Verification items for the finished model (mm, model axes). A direction names the side the tool comes from. Round coordinates to 2 decimals unless told otherwise and drop trailing zeros. Write each loop counter-clockwise with the first axis right and the second up, starting at its lowest first coordinate (ties: lowest second). Pieces come first, ordered by that corner, then holes. Notation, with made-up numbers: (-26.75, 80) -> (-1.75, 80) arc R36 cw to (-1.75, 119) -> close; hole circle Ø7 at (15.5, 23). An arc over 180 degrees is marked (long way). Answer as a JSON object with one key per item and string values. Group by question number.
(1) Scan lines: L1, parallel to X at y = -2.5, z = 265.5; L2, parallel to Z at x = 24, y = 9; L3, parallel to X at y = 18.5, z = 102. Record each from-to range of solid material in increasing order. Write a range as from..to.
(2) Set-up check for faces 1 (the face through (-5, -3.962, 267)), 2 (the face through (12.7, 0, 260)), 3 (the face through (-12.7, 0, 260)): record each of +Z, -Z, +X, -X, +Y, -Y from which the full face is reachable in a straight line by a thin tool's end or side.
(3) Sectioned sample at C-C on z = 104.5. Record the cut outline in (x, y), and give its area (3 significant figures).
(4) Sectioned sample at D-D on x = -15.5. Record the cut outline in (y, z), and give its area (3 significant figures).
(5) Sectioned sample at B-B on y = 0. Record the cut outline in (x, z).
(6) Gauge pin test, flat ends, axial feed: pin 1 Ø4 at (y, z) = (1, 262) entering from +X; pin 2 Ø3 at (y, z) = (11, 186) entering from +X; pin 3 Ø1.5 at (y, z) = (-1, 199.5) entering from +X. Record the tip position at first contact, or that the pin passes through.
(7) Sectioned sample at A-A on x = 0. Record the cut outline in (y, z), and give its area (3 significant figures).
(8) Draft check along X on faces 4 (the face through (5, 3.962, 267)), 5 (the face through (-0.279, 0.055, 279.397)), 6 (the face through (4.775, 0, 260)), 7 (the face through (-4.775, 0, 260)). Enter one of: released by +X, released by -X, zero draft, split by the parting line, or undercut.
Autodesk Inventor part; units mm, degrees
ref_plane "YZ Plane" through (0, 0, 0) normal (1, 0, 0) x (0, 1, 0)
ref_plane "XZ Plane" through (0, 0, 0) normal (0, 1, 0) x (-1, 0, 0)
ref_plane "XY Plane" through (0, 0, 0) normal (0, 0, 1) x (1, 0, 0)
sketch "Sketch1" plane through (0, 0, 0) normal (0, 0, 1) x (1, 0, 0)
  circle A0 centre (0, 0) radius 31.2674
  dimension "d0" = 62.5348
extrude "Extrusion1" add sketch "Sketch1" along normal blind 254
sketch "Sketch2" plane through (0, 0, 254) normal (0, 0, 1) x (1, 0, 0)
  circle A0 centre (0, 0) radius 31.2674
  line L0 (-12.7, 3.9624) -> (12.7, 3.9624)
  line L1 (12.7, 3.9624) -> (12.7, -3.9624)
  line L2 (12.7, -3.9624) -> (-12.7, -3.9624)
  line L3 (-12.7, -3.9624) -> (-12.7, 3.9624)
  dimension "d3" = 7.9248
  dimension "d4" = 3.9624
  dimension "d5" = 12.7
  dimension "d6" = 12.7
extrude "Extrusion2" add sketch "Sketch2" along normal blind 25.4 contours L0 L1 L2 L3
sketch "Sketch3" plane through (-12.7, 3.9624, 254) normal (0, 1, 0) x (1, 0, 0)
  line L0 (0, 0) -> (25.4, 0)
  line L1 (0, 0) -> (0, -25.4)
  line L2 (25.4, -25.4) -> (0, -25.4)
  line L3 (25.4, 0) -> (25.4, -25.4)
  arc A0 (0, -12.7) -> (25.4, -12.7) centre (12.7, -12.7) ccw
  line L4 (7.9248, 0) -> (7.9248, -12.7)
  line L5 (17.4752, 0) -> (17.4752, -12.7)
  arc A1 (7.9248, -12.7) -> (17.4752, -12.7) centre (12.7, -12.7) ccw
  point P0 (12.7, 254)
  dimension "d9" = 7.9248
extrude "Extrusion3" cut sketch "Sketch3" against normal blind 25.4 contours L0 L5 A1 L4 | A0 L2 L1 | A0 L3 L2
properties part number "Spring End"
Computed values:
{
 "1": {"L1": "-12.7..-4.78, 4.78..12.7", "L2": "0..254", "L3": "-25.21..25.21"},
 "2": {"face 1": "+Z, +X, -X, -Y", "face 2": "+Z, +X, +Y, -Y", "face 3": "+Z, -X, +Y, -Y"},
 "3": {"outline": "circle Ø62.53 at (0, 0)", "area": "3,070 mm2"},
 "4": {"outline": "(-27.16, 0) -> (27.16, 0) -> (27.16, 254) -> (-27.16, 254) -> close", "area": "13,800 mm2"},
 "5": {"outline": "(-31.27, 0) -> (31.27, 0) -> (31.27, 254) -> (12.7, 254) -> (12.7, 266.7) arc R12.7 ccw to (-12.7, 266.7) -> (-12.7, 254) -> (-31.27, 254) -> close; hole (-4.78, 254) -> (4.78, 254) -> (4.78, 266.7) arc R4.78 ccw to (-4.78, 266.7) -> close"},
 "6": {"pin 1": "x = 12.7", "pin 2": "x = 29.79", "pin 3": "x = 31.27"},
 "7": {"outline": "(-31.27, 0) -> (31.27, 0) -> (31.27, 254) -> (-31.27, 254) -> close; (-3.96, 271.48) -> (3.96, 271.48) -> (3.96, 279.4) -> (-3.96, 279.4) -> close", "area": "15,900 mm2"},
 "8": {"face 4": "zero draft", "face 5": "split by the parting line", "face 6": "undercut", "face 7": "undercut"}
}
